For this review, take the finished solid that the model builds, in its own axes (mm). Round coordinates to 2 decimals unless told otherwise and drop trailing zeros. Loops run counter-clockwise (first coordinate to the right, second up) from the corner with the lowest first, then second, coordinate; pieces in that order, holes last.
1) Take a section at B-B (z = 3.2). Give the number of separate pieces and of enclosed holes in the cut face, then the cut area to 3 significant figures.
2) Take a section at A-A (x = 147). State the section outline as (y, z) points, then the cut area to 3 significant figures.
3) Wall thickness on L1, parallel to Y at x = 115, z = 3.1; L2, parallel to Y at x = 55.5, z = 3.7; L3, parallel to X at y = -36, z = 3.55: over which ranges is each line inside the solid? List them lowest first.
4) Insertion check: pin 1 (3 mm diameter, centred on x = 305, y = -35.15, fed in from +Z); pin 2 (1.2 mm diameter, centred on x = 372.5, z = 2, fed in from +Y). Each pin has a flat end and moves straight along its axis. Give the tip position at first contact, or say it passes through.
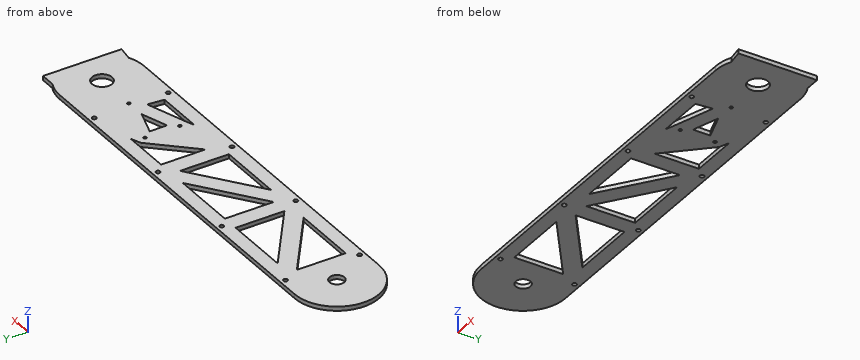
```python
from build123d import *

# Parameters (mm, degrees)
SKETCH_1_R          = 7.03
SKETCH_1_R_2        = 1.5
SKETCH_1_R_3        = 9.53
EXTRUDE_1_DEPTH     = 4
SKETCH_2_R          = 2
CUT_EXTRUDE_1_DEPTH = 10
CUT_EXTRUDE_4_DEPTH = 4
EXTRUDE_2_DEPTH     = 4


with BuildPart() as part:
    # 草图1 → 凸台-拉伸1 (new body)
    with BuildSketch(Plane.XY):
        with BuildLine():
            ThreePointArc((348.542857143, -40.145714286), (388.542857143, -0.145714286), (348.542857143, 39.854285714))
            Line((348.542857143, 39.854285714), (-1.457142857, 39.854285714))
            ThreePointArc((-1.457142857, 39.854285714), (-41.457142857, -0.145714286), (-1.457142857, -40.145714286))
            Line((-1.457142857, -40.145714286), (348.542857143, -40.145714286))
        make_face()
        with Locations((-1.457142857, -0.145714286)):
            Circle(SKETCH_1_R, mode=Mode.SUBTRACT)
        with Locations((258.542857143, -16.645714286)):
            Circle(SKETCH_1_R_2, mode=Mode.SUBTRACT)
        with Locations((258.542857143, 16.354285714)):
            Circle(SKETCH_1_R_2, mode=Mode.SUBTRACT)
        with Locations((308.542857143, -0.145714286)):
            Circle(SKETCH_1_R_2, mode=Mode.SUBTRACT)
        with Locations((348.542857143, -0.145714286)):
            Circle(SKETCH_1_R_3, mode=Mode.SUBTRACT)
    extrude(amount=EXTRUDE_1_DEPTH)

    # 草图2 → 切除-拉伸1 (cut)
    with BuildSketch(Plane.XY.offset(4)):
        Polygon((107, 26.854285714), (44.343341396, 26.854285714), (107, -19.31377852), align=None)
        Polygon((90.656658604, -27.145714286), (28, 19.022349949), (28, -27.145714286), align=None)
        with Locations((210, 34.854285714)):
            Circle(SKETCH_2_R)
        with Locations((115, -35.145714286)):
            Circle(SKETCH_2_R)
        Polygon((202, 19.022349949), (139.343341396, -27.145714286), (202, -27.145714286), align=None)
        Polygon((185.656658604, 26.854285714), (123, 26.854285714), (123, -19.31377852), align=None)
        Polygon((263.286571323, 26.854285714), (218, 26.854285714), (218, -14.994963043), (253.936816603, 23.131059281), align=None)
        Polygon((297.768914783, -27.145714286), (299.341875576, -11.606383875), (261.222229771, -24.18586699), (253.455773316, -27.145714286), align=None)
        Polygon((264.542857143, -8.347455032), (289.396616979, -0.145714286), (264.542857143, 8.05602646), align=None)
        with Locations((20, 34.854285714)):
            Circle(SKETCH_2_R)
        with Locations((115, 34.854285714)):
            Circle(SKETCH_2_R)
        with Locations((305, 34.854285714)):
            Circle(SKETCH_2_R)
        with Locations((305, -35.145714286)):
            Circle(SKETCH_2_R)
        with Locations((210, -35.145714286)):
            Circle(SKETCH_2_R)
        with Locations((20, -35.145714286)):
            Circle(SKETCH_2_R)
    extrude(amount=-CUT_EXTRUDE_1_DEPTH, mode=Mode.SUBTRACT)

    # 草图3 → 切除-拉伸4 (cut)
    with BuildSketch(Plane(origin=(0, 0, 0), x_dir=(-1, 0, 0), z_dir=(0, 0, -1))):
        Polygon((-379.542857143, -0.145714286), (-379.542857143, 86.711362621), (-469.13936256, 65.161980464), (-431.797169727, -71.622846313), (-379.542857143, -46.898899995), align=None)
    extrude(amount=-CUT_EXTRUDE_4_DEPTH, mode=Mode.SUBTRACT)

    # 草图4 → 凸台-拉伸2 (add)
    with BuildSketch(Plane(origin=(0, 0, 0), x_dir=(-1, 0, 0), z_dir=(0, 0, -1))):
        Polygon((-379.542857143, -25.424163605), (-379.542857143, -38.278889608), (-365.701849351, -36.278372455), (-365.701849351, 35.986943884), (-379.542857143, 35.986943884), (-379.542857143, 25.132735034), align=None)
    extrude(amount=-EXTRUDE_2_DEPTH)


solid = part.part
```
Response:
1. separate pieces: 1
1. enclosed holes: 20
1. area: 25,100 mm2
2. outline: (-40.15, 0) - (-27.15, 0) - (-27.15, 4) - (-40.15, 4) - close; (-21.5, 0) - (-1.63, 0) - (-1.63, 4) - (-21.5, 4) - close; (26.85, 0) - (39.85, 0) - (39.85, 4) - (26.85, 4) - close
2. area: 183 mm2
3. L1: y = -40.15 to -37.15, -33.15 to 32.85, 36.85 to 39.85
3. L2: y = -40.15 to -27.15, -1.24 to 18.63, 26.85 to 39.85
3. L3: x = -19.19 to 18.19, 21.81 to 113.19, 116.81 to 208.19, 211.81 to 303.19, 306.81 to 379.54
4. pin 1: passes through
4. pin 2: stops at y = 35.99
